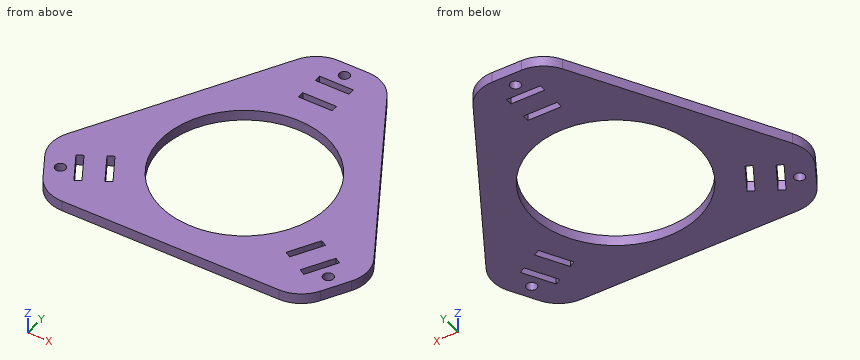
from build123d import *

# Parameters (mm, degrees)
SKETCH_1_R      = 1.5
SKETCH_1_R_2    = 24
SKETCH_1_W      = 9.7
SKETCH_1_H      = 1.95
EXTRUDE_4_DEPTH = 3


with BuildPart() as part:
    # Эскиз1 → Бобышка-Вытянуть4 (new body)
    with BuildSketch(Plane.XY):
        with BuildLine():
            Line((-31.207078757, -32.897754038), (31.207078757, -32.897754038))
            ThreePointArc((31.207078757, -32.897754038), (36.207078757, -31.558008076), (39.867332794, -27.897754038))
            Line((39.867332794, -27.897754038), (44.093830103, -20.577245962))
            ThreePointArc((44.093830103, -20.577245962), (45.433576065, -15.577245962), (44.093830103, -10.577245962))
            Line((44.093830103, -10.577245962), (12.886751346, 43.475))
            ThreePointArc((12.886751346, 43.475), (9.226497308, 47.135254038), (4.226497308, 48.475))
            Line((4.226497308, 48.475), (-4.226497308, 48.475))
            ThreePointArc((-4.226497308, 48.475), (-9.226497308, 47.135254038), (-12.886751346, 43.475))
            Line((-12.886751346, 43.475), (-44.093830103, -10.577245962))
            ThreePointArc((-44.093830103, -10.577245962), (-45.433576065, -15.577245962), (-44.093830103, -20.577245962))
            Line((-44.093830103, -20.577245962), (-39.867332794, -27.897754038))
            ThreePointArc((-39.867332794, -27.897754038), (-36.207078757, -31.558008076), (-31.207078757, -32.897754038))
        make_face()
        with Locations((-38.516479833, -22.2375)):
            Circle(SKETCH_1_R, mode=Mode.SUBTRACT)
        with Locations(Location((0, 44.475, 0), (0, 0, 180))):
            Circle(SKETCH_1_R, mode=Mode.SUBTRACT)
        with Locations((38.516479833, -22.2375)):
            Circle(SKETCH_1_R, mode=Mode.SUBTRACT)
        Circle(SKETCH_1_R_2, mode=Mode.SUBTRACT)
        Polygon((-33.06039092, -24.687723208), (-37.91039092, -16.287276792), (-36.221641383, -15.312276792), (-31.371641383, -23.712723208), align=None, mode=Mode.SUBTRACT)
        with Locations((0, 40)):
            Rectangle(SKETCH_1_W, SKETCH_1_H, mode=Mode.SUBTRACT)
        Polygon((37.91039092, -16.287276792), (33.06039092, -24.687723208), (31.371641383, -23.712723208), (36.221641383, -15.312276792), align=None, mode=Mode.SUBTRACT)
        Polygon((-26.565200392, -20.937723208), (-31.415200392, -12.537276792), (-29.726450854, -11.562276792), (-24.876450854, -19.962723208), align=None, mode=Mode.SUBTRACT)
        with Locations((0, 32.5)):
            Rectangle(SKETCH_1_W, SKETCH_1_H, mode=Mode.SUBTRACT)
        Polygon((31.415200392, -12.537276792), (26.565200392, -20.937723208), (24.876450854, -19.962723208), (29.726450854, -11.562276792), align=None, mode=Mode.SUBTRACT)
    extrude(amount=EXTRUDE_4_DEPTH)


solid = part.part
Could you check a few things on this model? Use its own coordinates, in mm. Give positions to 0.01 mm unless a question says otherwise; leave off trailing zeros. Write each loop counter-clockwise with the first axis right and the second up, starting at its lowest first coordinate (ties: lowest second). Pieces come first, ordered by that corner, then holes. Notation, with made-up numbers: (53, -29.5) -> (100, -29.5) arc R15 cw to (100, -13.5) -> close; hole circle Ø11 at (71.5, 24.25). An arc over 180 degrees is marked (long way). Answer as CSV lines item,"result". Start each with the question number.
(1) Please list where these lines run through material, in increasing order: line 1 (Y direction, x = 0, z = 2.25) (3 decimals); line 2 (X direction, y = -12, z = 2.6); line 3 (X direction, y = 13, z = 0.65).
(2) I'm going to push flat-ended pins straight in: pin 1 Ø2.5 at (x, y) = (38.52, -22.24) entering from -Z; pin 2 Ø0.6 at (y, z) = (40, 1.5) entering from +X; pin 3 Ø1 at (y, z) = (32.5, 1) entering from +X; pin 4 Ø1 at (x, y) = (0.5, 38) entering from -Z. Where does each tip first touch, or does it pass through?
(3) If we section it at B-B, the plane y = 0: Write out the boundary of the cut face in (x, z).
(4) If we section it at A-A, the plane x = 0: Write out the boundary of the cut face in (y, z) (3 decimals), and give its area (3 significant figures).
(5) If we section it at C-C, the plane z = 2.4: Give the number of separate pieces and of enclosed holes in the cut face, and give its area (3 significant figures).
Answer list:
1,line 1,"-32.898 to -24, 24 to 31.525, 33.475 to 39.025, 40.975 to 42.975, 45.975 to 48.475"
1,line 2,"-44.77 to -30.48, -29.47 to -20.78, 20.78 to 29.47, 30.48 to 44.77"
1,line 3,"-30.48 to -20.17, 20.17 to 30.48"
2,pin 1,"through"
2,pin 2,"x = 15.07"
2,pin 3,"x = 19.51"
2,pin 4,"z = 0"
3,outline,"(-37.99, 0) -> (-24, 0) -> (-24, 3) -> (-37.99, 3) -> close; (24, 0) -> (37.99, 0) -> (37.99, 3) -> (24, 3) -> close"
4,outline,"(-32.898, 0) -> (-24, 0) -> (-24, 3) -> (-32.898, 3) -> close; (24, 0) -> (31.525, 0) -> (31.525, 3) -> (24, 3) -> close; (33.475, 0) -> (39.025, 0) -> (39.025, 3) -> (33.475, 3) -> close; (40.975, 0) -> (42.975, 0) -> (42.975, 3) -> (40.975, 3) -> close; (45.975, 0) -> (48.475, 0) -> (48.475, 3) -> (45.975, 3) -> close"
4,area,"79.4 mm^2"
5,separate pieces,"1"
5,enclosed holes,"10"
5,area,"3,130 mm^2"
